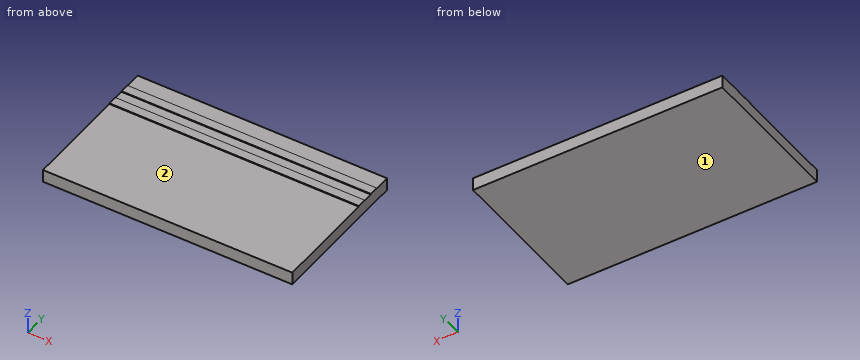
Autodesk Inventor part; units mm, degrees
ref_plane "YZ Plane" through (0, 0, 0) normal (1, 0, 0) x (0, 1, 0)
ref_plane "XZ Plane" through (0, 0, 0) normal (0, 1, 0) x (-1, 0, 0)
ref_plane "XY Plane" through (0, 0, 0) normal (0, 0, 1) x (1, 0, 0)
sketch "Skizze1" plane through (0, 0, 0) normal (0, 0, 1) x (1, 0, 0)
  line L0 (0, 0) -> (33, 0)
  line L1 (33, 0) -> (33, -19.5)
  line L2 (33, -19.5) -> (0, -19.5)
  line L3 (0, -19.5) -> (0, 0)
  dimension "d0" = 33
  dimension "d1" = 19.5
extrude "Extrusion1" add sketch "Skizze1" along normal blind 1.7
sketch "Skizze2" plane through (0, 0, 1.7) normal (0, 0, 1) x (1, 0, 0)
  line L0 (33, 0) -> (0, 0)
  line L1 (0, 0) -> (0, -19.5)
  line L2 (0, -19.5) -> (33, -19.5)
  line L3 (33, -19.5) -> (33, 0)
  line L4 (0, 0) -> (0, -19.5)
  line L5 (33, 0) -> (33, -19.5)
  line L6 (0, -2.15) -> (33, -2.15)
  line L7 (33, -2.15) -> (33, -3.35)
  line L8 (33, -3.35) -> (0, -3.35)
  line L9 (0, -3.35) -> (0, -2.15)
  line L10 (33, -5.85) -> (0, -5.85)
  line L11 (0, -5.85) -> (0, -4.65)
  line L12 (0, -4.65) -> (33, -4.65)
  line L13 (33, -4.65) -> (33, -5.85)
  line L14 (0, -3.35) -> (33, -3.35)
  line L15 (33, -3.35) -> (33, -2.15)
  line L16 (33, -2.15) -> (0, -2.15)
  line L17 (0, -2.15) -> (0, -3.35)
  line L18 (33, -4.65) -> (0, -4.65)
  line L19 (0, -4.65) -> (0, -5.85)
  line L20 (0, -5.85) -> (33, -5.85)
  line L21 (33, -5.85) -> (33, -4.65)
  dimension "d10" = 1.2
  dimension "d11" = 1.2
  dimension "d12" = 1.3
extrude "Extrusion2" add sketch "Skizze2" along normal blind 0.1 contours L3 L8 L1 L6 | L3 L10 L1 L12
sketch "Skizze4" plane through (0, 0, 1.7) normal (0, 0, 1) x (1, 0, 0)
  line L0 (429, -5.85) -> (0, -5.85)
  line L1 (0, -5.85) -> (0, -20)
  line L2 (0, -20) -> (429, -20)
  line L3 (429, -20) -> (429, -5.85)
  line L4 (0, -20) -> (-50, -20)
  line L5 (-50, -20) -> (-50, 20)
  line L6 (-50, 20) -> (0, 20)
  line L7 (0, 20) -> (0, -20)
  line L8 (23.5, 20) -> (11.5, 20)
  point P0 (0, 0)
  dimension "d19" = 50
sketch "Skizze5" plane through (0, 0, 1.7) normal (0, 0, 1) x (1, 0, 0)
  circle A0 centre (50.5, 14) radius 1.5
  circle A1 centre (83.5, 14) radius 1.5
  circle A2 centre (116.5, 14) radius 1.5
  circle A3 centre (149.5, 14) radius 1.5
  circle A4 centre (182.5, 14) radius 1.5
  circle A5 centre (215.5, 14) radius 1.5
  circle A6 centre (248.5, 14) radius 1.5
  circle A7 centre (281.5, 14) radius 1.5
  circle A8 centre (314.5, 14) radius 1.5
  circle A9 centre (347.5, 14) radius 1.5
  circle A10 centre (380.5, 14) radius 1.5
  circle A11 centre (413.5, 14) radius 1.5
  circle A12 centre (17.5, 14) radius 1.5
  line L0 (0, -2.15) -> (429, -2.15)
  line L1 (429, -2.15) -> (429, 0)
  line L2 (429, 0) -> (419.5, 0)
  line L3 (419.5, 0) -> (419.5, 20)
  line L4 (419.5, 20) -> (407.5, 20)
  line L5 (407.5, 20) -> (407.5, 0)
  line L6 (407.5, 0) -> (386.5, 0)
  line L7 (386.5, 0) -> (386.5, 20)
  line L8 (386.5, 20) -> (374.5, 20)
  line L9 (374.5, 20) -> (374.5, 0)
  line L10 (374.5, 0) -> (353.5, 0)
  line L11 (353.5, 0) -> (353.5, 20)
  line L12 (353.5, 20) -> (341.5, 20)
  line L13 (341.5, 20) -> (341.5, 0)
  line L14 (341.5, 0) -> (320.5, 0)
  line L15 (320.5, 0) -> (320.5, 20)
  line L16 (320.5, 20) -> (308.5, 20)
  line L17 (308.5, 20) -> (308.5, 0)
  line L18 (308.5, 0) -> (287.5, 0)
  line L19 (287.5, 0) -> (287.5, 20)
  line L20 (287.5, 20) -> (275.5, 20)
  line L21 (275.5, 20) -> (275.5, 0)
  line L22 (275.5, 0) -> (254.5, 0)
  line L23 (254.5, 0) -> (254.5, 20)
  line L24 (254.5, 20) -> (242.5, 20)
  line L25 (242.5, 20) -> (242.5, 0)
  line L26 (242.5, 0) -> (221.5, 0)
  line L27 (221.5, 0) -> (221.5, 20)
  line L28 (221.5, 20) -> (209.5, 20)
  line L29 (209.5, 20) -> (209.5, 0)
  line L30 (209.5, 0) -> (188.5, 0)
  line L31 (188.5, 0) -> (188.5, 20)
  line L32 (188.5, 20) -> (176.5, 20)
  line L33 (176.5, 20) -> (176.5, 0)
  line L34 (176.5, 0) -> (155.5, 0)
  line L35 (155.5, 0) -> (155.5, 20)
  line L36 (155.5, 20) -> (143.5, 20)
  line L37 (143.5, 20) -> (143.5, 0)
  line L38 (143.5, 0) -> (122.5, 0)
  line L39 (122.5, 0) -> (122.5, 20)
  line L40 (122.5, 20) -> (110.5, 20)
  line L41 (110.5, 20) -> (110.5, 0)
  line L42 (110.5, 0) -> (89.5, 0)
  line L43 (89.5, 0) -> (89.5, 20)
  line L44 (89.5, 20) -> (77.5, 20)
  line L45 (77.5, 20) -> (77.5, 0)
  line L46 (77.5, 0) -> (56.5, 0)
  line L47 (56.5, 0) -> (56.5, 20)
  line L48 (56.5, 20) -> (44.5, 20)
  line L49 (44.5, 20) -> (44.5, 0)
  line L50 (44.5, 0) -> (23.5, 0)
  line L51 (23.5, 0) -> (23.5, 20)
  line L52 (23.5, 20) -> (11.5, 20)
  line L53 (11.5, 20) -> (11.5, 0)
  line L54 (11.5, 0) -> (0, 0)
  line L55 (0, 0) -> (0, 20)
  line L56 (0, 20) -> (-50, 20)
  line L57 (-50, 20) -> (-50, -20)
  line L58 (-50, -20) -> (429, -20)
  line L59 (429, -20) -> (429, -5.85)
  line L60 (429, -5.85) -> (0, -5.85)
  line L61 (0, -4.65) -> (0, -5.85)
  line L62 (0, -4.65) -> (429, -4.65)
  line L63 (429, -4.65) -> (429, -3.35)
  line L64 (429, -3.35) -> (0, -3.35)
  line L65 (0, -2.15) -> (0, -3.35)
  line L66 (-38.9172, -16.707) -> (-48.9487, -16.707)
  line L67 (-48.9487, -16.707) -> (-48.9487, -8.753)
  line L68 (-48.9487, -8.753) -> (-38.9172, -8.753)
  line L69 (-38.9172, -8.753) -> (-38.9172, -16.707)
  line L70 (-40.6386, -6.9723) -> (-48.9487, -6.9723)
  line L71 (-48.9487, -6.9723) -> (-48.9487, -2.75)
  line L72 (-48.9487, -2.75) -> (-40.6386, -2.75)
  line L73 (-40.6386, -2.75) -> (-40.6386, -6.9723)
sketch "Skizze6" plane through (0, 0, 1.7) normal (0, 0, 1) x (1, 0, 0)
  circle A0 centre (-40.9672, 3.5952) radius 2
  point P0 (0, 0)
  dimension "d25" = 4
  dimension "d29" = 20
  dimension "d30" = 1.3
  dimension "d31" = 1.2
  dimension "d32" = 1.2
  dimension "d33" = 2.15
properties part number "PowerRail"
The model under review builds one solid part; all positions refer to its coordinate system, in mm. Face numbers are marked on the shaded views. A direction names the side the tool comes from. Coordinates: 2 decimals unless noted, no trailing zeros. Write each loop counter-clockwise with the first axis right and the second up, starting at its lowest first coordinate (ties: lowest second). Pieces come first, ordered by that corner, then holes. Notation, with made-up numbers: (7.5, 15.5) - (27.5, 15.5) arc R25 cw to (27.5, 39.5) - close; hole circle Ø1 at (-7.75, 30.25). An arc over 180 degrees is marked (long way). Answer as a JSON object with one key per item and string values. Group by question number.
1. Machinability: for the marked faces 1 and 2, which of the approach directions +Z, -Z, +X, -X, +Y, -Y give a long, thin tool a straight path to every point of the face, cutting with its end or side? Answer none if there is none.
2. Add section B-B (y = -13.25). Give the boundary of the cut face in (x, z).
3. Add section A-A (x = 15.5). Give the boundary of the cut face in (y, z), plus the area to 3 significant figures.
4. Clearance check with a flat-ended pin moving along its axis: pin 1 Ø11 at (x, y) = (10, -14.5) entering from +Z. State where the tip first meets the part, or that it passes through.
5. To check wall thickness, follow probe 1 along Z at (x, y) = (11, -18.5). State the ranges of the line that lie inside material, in increasing order.
Findings:
{
 "1": {"face 1": "-Z, +X, -X, +Y, -Y", "face 2": "+Z, +X, -X, -Y"},
 "2": {"outline": "(0, 0) - (33, 0) - (33, 1.7) - (0, 1.7) - close"},
 "3": {"outline": "(-19.5, 0) - (0, 0) - (0, 1.7) - (-2.15, 1.7) - (-2.15, 1.8) - (-3.35, 1.8) - (-3.35, 1.7) - (-4.65, 1.7) - (-4.65, 1.8) - (-5.85, 1.8) - (-5.85, 1.7) - (-19.5, 1.7) - close", "area": "33.4 mm²"},
 "4": {"pin 1": "z = 1.7"},
 "5": {"probe 1": "0 to 1.7"}
}
